from build123d import *

# Parameters (mm, degrees)
F3_SIZE         = 0.254
F4_W            = 0.508
F4_H            = 3.048
F6_DEPTH        = 4.572
F6_COPIES_COUNT = 6
F7_R            = 0.127
F8_R            = 0.0508


# Not quite as in the source:
# - a pattern or mirror of a feature is missing from the dataset's text; its kind, count and spacing are read off the source's solid


with BuildPart() as f1:
    # F0 (on Front) → F1 (revolve)
    with BuildSketch(Plane.XZ):
        with BuildLine():
            Line((2.2098, 0), (2.8448, 0))
            Line((2.8448, 0), (2.8448, 4.572))
            Line((2.8448, 4.572), (2.7178, 4.572))
            Line((2.7178, 4.572), (2.7178, 7.1363093255))
            Line((2.7178, 7.1363093255), (2.2479, 8.89))
            Line((2.2479, 8.89), (2.2479, 1.397))
            ThreePointArc((2.2479, 1.397), (2.2107025612, 1.3071974388), (2.1209, 1.27))
            Line((2.1209, 1.27), (0, 1.27))
            Line((0, 1.27), (0, 0.3969097134))
            ThreePointArc((0, 0.3969097134), (1.1225811063, 0.2968946462), (2.2098, 0))
        make_face()
    revolve(axis=Axis((0, 0, 7.5646454352), (0, 0, 1)))

    # F3
    f3_edges = [f1.edges().sort_by_distance(p)[0] for p in [
        (-2.8448, 0, 0),
    ]]
    chamfer(f3_edges, length=F3_SIZE)

    # F4 (on offset) → F6 (cut)
    with BuildSketch(Plane.XY.offset(8.89)):
        with Locations((0, 1.524)):
            Rectangle(F4_W, F4_H)
    f6 = extrude(amount=-F6_DEPTH, mode=Mode.SUBTRACT)

    # F6_copies: F6 ×6 about axis
    f6_copies_axis = Axis((0, 0, 0), (0, 0, 1))
    for i in range(1, F6_COPIES_COUNT):
        add(f6.rotate(f6_copies_axis, i * 360 / F6_COPIES_COUNT), mode=Mode.SUBTRACT)

    # F7
    f7_edges = [f1.edges().sort_by_distance(p)[0] for p in [
        (-0.254, 2.533471, 4.318),
        (0.254, 2.533471, 4.318),
        (2.32105, 1.046765, 4.318),
        (2.06705, 1.486706, 4.318),
        (-2.06705, 1.486706, 4.318),
        (-2.32105, 1.046765, 4.318),
        (-2.32105, -1.046765, 4.318),
        (-2.06705, -1.486706, 4.318),
        (-0.254, -2.533471, 4.318),
        (0.254, -2.533471, 4.318),
        (2.06705, -1.486706, 4.318),
        (2.32105, -1.046765, 4.318),
    ]]
    fillet(f7_edges, radius=F7_R)

    # F8
    f8_edges = [f1.edges().sort_by_distance(p)[0] for p in [
        (2.7178, 0, 4.572),
        (1.3589, 2.353684, 4.572),
        (-1.3589, 2.353684, 4.572),
        (1.3589, -2.353684, 4.572),
        (-2.7178, 0, 4.572),
        (-1.3589, -2.353684, 4.572),
    ]]
    fillet(f8_edges, radius=F8_R)


solid = f1.part
CAD build for the part. Positions are in the model's coordinates, mm. A direction names the side the tool comes from. Coordinates: 2 decimals unless noted, no trailing zeros. Loops run counter-clockwise (first coordinate to the right, second up) from the corner with the lowest first, then second, coordinate; pieces in that order, holes last. Notation, with made-up numbers: (-36.5, 37) -> (-29.5, 37) arc R19 cw to (-29.5, 57) -> close; hole circle Ø8 at (-2, 74). An arc over 180 degrees is marked (long way). One line per item, written item: value.
1. Slice it at C-C on y = 0. Write the cut outline in (x, z).
Answers:
outline: (-2.84, 0.25) -> (-2.59, 0) -> (-2.21, 0) arc R6.35 cw to (2.21, 0) -> (2.59, 0) -> (2.84, 0.25) -> (2.84, 4.57) -> (2.77, 4.57) arc R0.05 cw to (2.72, 4.62) -> (2.72, 7.14) -> (2.25, 8.89) -> (2.25, 1.4) arc R0.13 cw to (2.12, 1.27) -> (-2.12, 1.27) arc R0.13 cw to (-2.25, 1.4) -> (-2.25, 8.89) -> (-2.72, 7.14) -> (-2.72, 4.62) arc R0.05 cw to (-2.77, 4.57) -> (-2.84, 4.57) -> close
2. Flat gauge pin, fed straight in: P1, Ø2, axis at y = -2.5, z = 7, coming from the +X side. Where does the tip first touch, or does it go through?
Answers:
P1: stops at x = 2.22
3. Pull direction Y, two halves, no side cores. Call faces 4 (the face through (1.23, -2.15, 8.03)), 5 (the face through (1.037, -1.994, 5.091)), 6 (the face through (-1.345, 2.362, 5.897)): pulls with the +Y half, pulls with the -Y half, needs draft (parallel to the pull), parting line crosses it, or undercut.
Answers:
face 4: pulls with the -Y half
face 5: undercut
face 6: pulls with the +Y half
4. Slice it at D-D on z = 1.5. Write the cut outline in (x, y).
Answers:
outline: circle Ø5.69 at (0, 0); hole circle Ø4.5 at (0, 0)
5. Slice it at A-A on z = 7. Write the cut outline in (x, y).
Answers:
outline: (-2.47, -1.13) -> (-2.06, -0.9) arc R2.25 cw to (-2.06, 0.9) -> (-2.47, 1.13) arc R2.72 ccw to start; (-2.22, -1.57) arc R2.72 ccw to (-0.25, -2.71) -> (-0.25, -2.23) arc R2.25 cw to (-1.81, -1.34) -> close; (-2.22, 1.57) -> (-1.81, 1.34) arc R2.25 cw to (-0.25, 2.23) -> (-0.25, 2.71) arc R2.72 ccw to start; (0.25, -2.71) arc R2.72 ccw to (2.22, -1.57) -> (1.81, -1.34) arc R2.25 cw to (0.25, -2.23) -> close; (0.25, 2.23) arc R2.25 cw to (1.81, 1.34) -> (2.22, 1.57) arc R2.72 ccw to (0.25, 2.71) -> close; (2.06, -0.9) -> (2.47, -1.13) arc R2.72 ccw to (2.47, 1.13) -> (2.06, 0.9) arc R2.25 cw to start
6. Which spindle directions (+Z, -Z, +X, -X, +Y, -Y) get a long thin tool onto all of the face, cutting with end or side? Do faces 1 (the face through (-1.373, -2.345, 5.897)), 2 (the face through (1.345, -2.362, 5.897)), 3 (the face through (2.718, -0.016, 5.897)). Say none if no direction does.
Answers:
face 1: +Z, -X, -Y
face 2: +Z, +X, -Y
face 3: +Z, +X
7. Slice it at B-B on x = 0. Write the cut outline in (y, z), and give its area (3 significant figures).
Answers:
outline: (-2.84, 0.25) -> (-2.59, 0) -> (-2.21, 0) arc R6.35 cw to (2.21, 0) -> (2.59, 0) -> (2.84, 0.25) -> (2.84, 4.32) -> (2.25, 4.32) -> (2.25, 1.4) arc R0.13 cw to (2.12, 1.27) -> (-2.12, 1.27) arc R0.13 cw to (-2.25, 1.4) -> (-2.25, 4.32) -> (-2.84, 4.32) -> close
area: 9.63 mm^2
8. Drill centre lines: line 1 (X direction, y = 1.9, z = 3.75); line 2 (Y direction, x = -1.5, z = 7.75); line 3 (Y direction, x = 0.65, z = 3.75). Where is each one in solid material? Low to high. Write a range as [from, to].
Answers:
line 1: x = [-2.12, -1.2], [1.2, 2.12]
line 2: y = [-2.07, -1.67], [1.67, 2.07]
line 3: y = [-2.77, -2.15], [2.15, 2.77]
